The model under review builds one solid part; all positions refer to its coordinate system, in mm. Face numbers are marked on the shaded views. A direction names the side the tool comes from. Coordinates: 2 decimals unless noted, no trailing zeros. Loops run counter-clockwise (first coordinate to the right, second up) from the corner with the lowest first, then second, coordinate; pieces in that order, holes last. Notation, with made-up numbers: M 88.25,2.25 L 139.25,2.25 A18 cw 139.25,34.25 Z; hole C -0.75,48.25 d1. An arc over 180 degrees is marked long. Use CSV: the item, a comma, the result in double quotes. Start each with the question number.
1. Add section D-D, the plane x = 14. Write out the cut boundary in (y, z), then the cut area to 3 significant figures.
2. Add section C-C, the plane y = 5.75. Write out the cut boundary in (x, z).
3. Tool access review of the marked faces 4 and 5: name each direction out of +Z, -Z, +X, -X, +Y, -Y from which nothing blocks a thin tool from reaching the whole face with its end or side.
4. Clearance check with flat-ended pins moving along their axes: P1, Ø6, axis at y = 2.5, z = 68.5, coming from the -X side; P2, Ø20, axis at x = 27.5, z = 71, coming from the +Y side; P3, Ø1.1, axis at x = 41.5, z = 60.5, coming from the +Y side; P4, Ø15, axis at x = 28, z = 29.5, coming from the +Y side. State where each tip first meets the part, or that it passes through.
5. Add section B-B, the plane z = 51.5. Write out the cut boundary in (x, y), then the cut area to 3 significant figures.
6. Draft analysis for pull direction X (two halves, no side actions). For the marked faces 1, 2 and 3, state which applies: +X half, -X half, draft (parallel to the pull), parting line (faces both ways), or undercut.
7. Add section A-A, the plane y = 16. Write out the cut boundary in (x, z), then the cut area to 3 significant figures.
8. For L1, parallel to Z at x = 30, y = 10.25; L2, parallel to X at y = 11.5, z = 12; L3, parallel to Z at x = 16, y = 12.25, list the stretches that pass through material, from the lowest coordinate up.
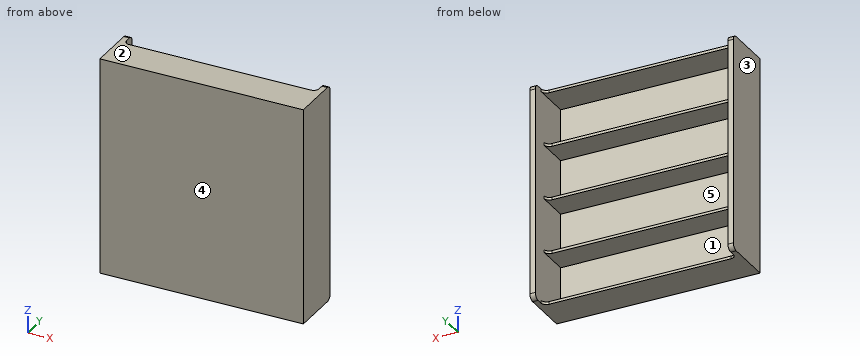
Autodesk Inventor part; units mm, degrees
ref_plane "YZ Plane" through (0, 0, 0) normal (1, 0, 0) x (0, 1, 0)
ref_plane "XZ Plane" through (0, 0, 0) normal (0, 1, 0) x (-1, 0, 0)
ref_plane "XY Plane" through (0, 0, 0) normal (0, 0, 1) x (1, 0, 0)
sketch "Эскиз1" plane through (0, 0, 0) normal (0, 1, 0) x (-1, 0, 0)
  line L0 (0, 0) -> (-75, 0)
  line L1 (-75, 0) -> (-75, 80)
  line L2 (-75, 80) -> (0, 80)
  line L3 (0, 80) -> (0, 0)
  line L4 (0, 60) -> (-75, 60)
  line L5 (0, 61) -> (-75, 61)
  line L6 (0, 79) -> (-75, 79)
  line L7 (0, 40) -> (-75, 40)
  line L8 (-75, 20) -> (0, 20)
  line L9 (0, 1) -> (-75, 1)
  line L10 (0, 21) -> (-75, 21)
  line L11 (0, 41) -> (-75, 41)
  line L12 (-2, 80) -> (-2, 0)
  line L13 (-73, 0) -> (-73, 80)
  point P0 (-73, 20)
  point P1 (-73, 1)
  point P2 (-2, 1)
  point P3 (-2, 20)
  point P4 (-73, 40)
  point P5 (-73, 21)
  point P6 (-2, 21)
  point P7 (-2, 40)
  point P8 (-73, 60)
  point P9 (-73, 41)
  point P10 (-2, 41)
  point P11 (-2, 60)
  point P12 (-73, 79)
  point P13 (-73, 61)
  point P14 (-2, 61)
  point P15 (-2, 79)
  dimension "d0" = 75
  dimension "d1" = 80
  dimension "d2" = 20
  dimension "d3" = 1
  dimension "d4" = 1
  dimension "d5" = 20
  dimension "d6" = 20
  dimension "d7" = 19
  dimension "d8" = 1
  dimension "d9" = 1
  dimension "d10" = 2
  dimension "d11" = 2
extrude "Выдавливание1" add sketch "Эскиз1" along normal blind 1 contours L9 L13 L8 L12 | L10 L13 L7 L12 | L11 L13 L4 L12 | L5 L13 L6 L12
extrude "Выдавливание2" add sketch "Эскиз1" along normal blind 19 contours L0 L12 L9 L3 | L9 L12 L8 L3 | L0 L1 L9 L13 | L8 L12 L10 L3 | L9 L1 L8 L13 | L10 L12 L7 L3 | L8 L1 L10 L13 | L7 L12 L11 L3 | L10 L1 L7 L13 | L11 L12 L4 L3 | L7 L1 L11 L13 | L4 L12 L5 L3 | L11 L1 L4 L13 | L5 L12 L6 L3 | L4 L1 L5 L13 | L6 L12 L2 L3 | L5 L1 L6 L13 | L6 L1 L2 L13
extrude "Выдавливание3" add sketch "Эскиз1" along normal blind 13 contours L0 L13 L9 L12 | L6 L13 L2 L12
extrude "Выдавливание4" add sketch "Эскиз1" along normal blind 11 contours L8 L13 L10 L12 | L7 L13 L11 L12 | L4 L13 L5 L12
fillet "Сопряжение1" radius 2 4 edges at (1, 19, 80) (1, 19, 0) (74, 19, 0) (74, 19, 80)
fillet "Сопряжение2" radius 2 10 edges at (2, 13, 79.5) (2, 11, 20.5) (2, 11, 40.5) (2, 11, 60.5) (2, 13, 0.5) (73, 13, 0.5) (73, 11, 20.5) (73, 11, 40.5) (73, 11, 60.5) (73, 13, 79.5)
properties part number "BatteryCompartment"
Computed:
1,outline,"M 0,0 L 13,0 L 13,1 L 1,1 L 1,20 L 11,20 L 11,21 L 1,21 L 1,40 L 11,40 L 11,41 L 1,41 L 1,60 L 11,60 L 11,61 L 1,61 L 1,79 L 13,79 L 13,80 L 0,80 Z"
1,area,"134 mm^2"
2,outline,"M 0,0 L 75,0 L 75,80 L 0,80 Z; hole M 2,1 L 73,1 L 73,20 L 2,20 Z; hole M 2,21 L 73,21 L 73,40 L 2,40 Z; hole M 2,41 L 73,41 L 73,60 L 2,60 Z; hole M 2,61 L 73,61 L 73,79 L 2,79 Z"
3,face 4,"+Z, -Z, +X, -X, -Y"
3,face 5,"+Y"
4,P1,"stops at x = 0"
4,P2,"stops at y = 13"
4,P3,"stops at y = 11"
4,P4,"stops at y = 1"
5,outline,"M 0,0 L 75,0 L 75,19 L 73,19 L 73,1 L 2,1 L 2,19 L 0,19 Z"
5,area,"147 mm^2"
6,face 1,"undercut"
6,face 2,"draft"
6,face 3,"-X half"
7,outline,"M 0,0 L 2,0 L 2,80 L 0,80 Z; M 73,0 L 75,0 L 75,80 L 73,80 Z"
7,area,"320 mm^2"
8,L1,"z = 0 to 1, 20 to 21, 40 to 41, 60 to 61, 79 to 80"
8,L2,"x = 0 to 2, 73 to 75"
8,L3,"z = 0 to 1, 79 to 80"
